Can you work these out from the model? Positions are in its coordinate system, mm. Give positions to 0.01 mm unless a question says otherwise; leave off trailing zeros. Order: outer loops, then holes, each group sorted by start corner. A loop starts at its lowest first (then second) coordinate and runs counter-clockwise, first axis right, second up.
Item 1: If I drill on line 1 along X through (y, z) = (2.25, 101.6); line 2 along X through (y, z) = (4.25, 222); line 3 along X through (y, z) = (2.5, 116.5), over which ranges is the centre line in solid material (lowest first)?
Item 2: I want a section at B-B, the plane y = 2.2. Write out the boundary of the cut face in (x, z), then the cut area to 3 significant figures.
Item 3: I want a section at A-A, the plane z = 101.6. Write out the boundary of the cut face in (x, y), then the cut area to 3 significant figures.
Item 4: I'm going to push flat-ended pins straight in: pin 1 Ø1.4 at (y, z) = (5.5, 125) entering from -X; pin 2 Ø0.6 at (y, z) = (5.5, 123) entering from +X; pin 3 Ø1.4 at (y, z) = (5.5, 124.5) entering from +X; pin 4 Ø9 at (x, z) = (0, 101.6) entering from +Y. Where does each tip first touch, or does it pass through?
Item 5: If we mould it in two halves opening along Z, with no side actions, what happens to faces 1 (the flat face through (1, 0, 175)), 2 (the flat face through (6, 4.724, 121)), 3 (the flat face through (-1, 3, 0))? For each: +Z half, -Z half, draft (parallel to the pull), parting line (faces both ways), or undercut.
Item 6: I want a section at D-D, the plane z = 243. Write out the boundary of the cut face in (x, y).
Item 7: I want a section at C-C, the plane z = 174.5. Write out the boundary of the cut face in (x, y), then the cut area to 3 significant figures.
```python
from build123d import *

# Parameters (mm, degrees)
BOSS_EXTRUDE1_DEPTH = 5.9944
SKETCH2_R           = 5.08
CUT_EXTRUDE1_DEPTH  = 368.170623747
CUT_EXTRUDE2_DEPTH  = 1.27
FILLET1_R           = 6.35


with BuildPart() as part:
    # Sketch1 → Boss-Extrude1 (new body)
    with BuildSketch(Plane(origin=(0, 0, 0), x_dir=(1, 0, 0), z_dir=(0, 1, 0))):
        Polygon((-67.945, 0), (67.945, 0), (91.252255377, -355.6), (-91.252255377, -355.6), align=None)
    extrude(amount=BOSS_EXTRUDE1_DEPTH)

    # Sketch2 → Cut-Extrude1 (cut, through all)
    with BuildSketch(Plane(origin=(0, 5.9944, 0), x_dir=(1, 0, 0), z_dir=(0, 1, 0))):
        with Locations(Location((0, -101.6, 0), (0, 0, 270))):
            Circle(SKETCH2_R)
    extrude(amount=-CUT_EXTRUDE1_DEPTH, mode=Mode.SUBTRACT)

    # Sketch3 → Cut-Extrude2 (cut)
    # profile 1 of 2: a face of its own
    with BuildSketch(Plane(origin=(0, 5.9944, 0), x_dir=(1, 0, 0), z_dir=(0, 1, 0))):
        Polygon((-0.64745098, -123.339411765), (-2.041960784, -123.339411765), (-2.041960784, -125.73), (-2.838823529, -125.73), (-2.838823529, -123.339411765), (-7.420784314, -123.339411765), (-7.420784314, -122.54254902), (-2.676960784, -115.769215686), (-2.041960784, -115.769215686), (-2.041960784, -122.54254902), (-0.64745098, -122.54254902), align=None)
        Polygon((-2.838823529, -122.54254902), (-2.838823529, -117.185514706), (-6.589681373, -122.54254902), align=None, mode=Mode.SUBTRACT)
    # profile 2 of 2: a face of its own
    with BuildSketch(Plane(origin=(0, 5.9944, 0), x_dir=(1, 0, 0), z_dir=(0, 1, 0))):
        with BuildLine():
            add(Edge.make_bspline(
                [(2.583578431, -120.288921569), (2.469757768, -120.233881465), (2.249012298, -120.12713588), (1.956518664, -119.921342429), (1.702152679, -119.699076506), (1.501146738, -119.44377738), (1.338617892, -119.168616459), (1.228149162, -118.865639865), (1.155782886, -118.539856671), (1.148992832, -118.313778727), (1.145490196, -118.197156863)],
                knots=[0, 0, 0, 0, 1.121505956, 2.175065151, 3.167266929, 4.111724904, 5.049364576, 5.994542137, 6.965488487, 8, 8, 8, 8], degree=3))
            add(Edge.make_bspline(
                [(1.145490196, -118.197156863), (1.150650446, -118.072365116), (1.160750204, -117.828119903), (1.228851738, -117.472785505), (1.349283719, -117.141800757), (1.514672213, -116.835914328), (1.722446411, -116.558323216), (1.961706137, -116.307792449), (2.237618257, -116.091502351), (2.542166789, -115.903299875), (2.878819269, -115.755673627), (3.240549794, -115.643784068), (3.628448984, -115.583063263), (3.894888198, -115.574417097), (4.031004902, -115.57)],
                knots=[0, 0, 0, 0, 1.029797524, 2.015542871, 2.97168719, 3.925682005, 4.874436321, 5.825197768, 6.775997772, 7.759919145, 8.771905717, 9.801204739, 10.876694018, 12, 12, 12, 12], degree=3))
            add(Edge.make_bspline(
                [(4.031004902, -115.57), (4.168265453, -115.573915681), (4.437144184, -115.581586081), (4.826482227, -115.649360813), (5.193306386, -115.752803643), (5.528540282, -115.908692567), (5.837903626, -116.092702905), (6.1102298, -116.31471085), (6.35377186, -116.560126292), (6.554706316, -116.839931798), (6.724312123, -117.141452673), (6.837039409, -117.474041466), (6.912766198, -117.827458116), (6.919373101, -118.072230943), (6.922745098, -118.197156863)],
                knots=[0, 0, 0, 0, 1.129990317, 2.213530109, 3.246876235, 4.260696229, 5.250296002, 6.204863837, 7.14791721, 8.090040244, 9.034951547, 9.986644228, 10.972433637, 12, 12, 12, 12], degree=3))
            add(Edge.make_bspline(
                [(6.922745098, -118.197156863), (6.919216595, -118.313762788), (6.912376396, -118.539809833), (6.840365414, -118.865811955), (6.728782095, -119.16750517), (6.571087227, -119.445784939), (6.365570739, -119.697892228), (6.112007529, -119.921560928), (5.819142842, -120.127075675), (5.598450258, -120.233860983), (5.484656863, -120.288921569)],
                knots=[0, 0, 0, 0, 1.034356649, 2.00515765, 2.950193721, 3.883105322, 4.833207204, 5.825260452, 6.878661931, 8, 8, 8, 8], degree=3))
            add(Edge.make_bspline(
                [(5.484656863, -120.288921569), (5.629584904, -120.345274008), (5.909015189, -120.453925018), (6.287487251, -120.674211509), (6.609031926, -120.93355376), (6.873327893, -121.233567804), (7.075041903, -121.576427985), (7.218061472, -121.958672451), (7.307398658, -122.379704945), (7.316483523, -122.673858557), (7.321176471, -122.825808824)],
                knots=[0, 0, 0, 0, 1.104307536, 2.129173671, 3.099289652, 4.029922044, 4.956040619, 5.91100379, 6.920891952, 8, 8, 8, 8], degree=3))
            add(Edge.make_bspline(
                [(7.321176471, -122.825808824), (7.318321613, -122.949426035), (7.312758231, -123.190324178), (7.265802022, -123.539824084), (7.187729342, -123.864910338), (7.08225254, -124.169001718), (6.941227364, -124.448040534), (6.773245337, -124.7078841), (6.567526726, -124.937879056), (6.337999195, -125.1468091), (6.085093931, -125.326864216), (5.825207776, -125.49131202), (5.550637227, -125.624540533), (5.268662499, -125.738439853), (4.972715633, -125.821171296), (4.668146304, -125.883957252), (4.352586022, -125.922213573), (4.139017278, -125.926863823), (4.031004902, -125.929215686)],
                knots=[0, 0, 0, 0, 1.165158113, 2.270593413, 3.316967265, 4.313258111, 5.297614584, 6.258105811, 7.221631145, 8.198179015, 9.17849254, 10.144943439, 11.094310651, 12.051658199, 13.00840578, 13.986862741, 14.981855988, 16, 16, 16, 16], degree=3))
            add(Edge.make_bspline(
                [(4.031004902, -125.929215686), (3.875058258, -125.925696781), (3.571935445, -125.918856875), (3.134122695, -125.846848764), (2.72518677, -125.740751294), (2.34901118, -125.583969435), (2.003278658, -125.380987257), (1.698555205, -125.12058817), (1.419046499, -124.819504607), (1.183989068, -124.46822424), (0.986969857, -124.087207102), (0.851225779, -123.680518964), (0.762222762, -123.259231693), (0.752157029, -122.971528144), (0.747058824, -122.825808824)],
                knots=[0, 0, 0, 0, 1.105131574, 2.1481103, 3.138917951, 4.095657432, 5.029651657, 5.970060793, 6.928497124, 7.934844507, 8.958454957, 9.961540876, 10.967538361, 12, 12, 12, 12], degree=3))
            add(Edge.make_bspline(
                [(0.747058824, -122.825808824), (0.750958552, -122.681150729), (0.75854413, -122.399768191), (0.842695471, -121.995459368), (0.973276047, -121.622346822), (1.158365157, -121.279786493), (1.410049218, -120.969502557), (1.737856358, -120.703220915), (2.131081537, -120.465798713), (2.427881476, -120.34978217), (2.583578431, -120.288921569)],
                knots=[0, 0, 0, 0, 1.026535231, 1.996771007, 2.920245165, 3.827596735, 4.74995178, 5.739273443, 6.81405554, 8, 8, 8, 8], degree=3))
        make_face()
        with BuildLine():
            add(Edge.make_bspline(
                [(6.125882353, -118.228284314), (6.123712551, -118.138717354), (6.119482737, -117.964115492), (6.062504916, -117.712266336), (5.98038969, -117.47610598), (5.859680999, -117.260408538), (5.712107035, -117.063654994), (5.541353334, -116.884667003), (5.342009506, -116.731408764), (5.12047127, -116.600704242), (4.877544231, -116.494065356), (4.612645581, -116.419299497), (4.328142503, -116.37607471), (4.131800472, -116.369987645), (4.031004902, -116.366862745)],
                knots=[0, 0, 0, 0, 1.025357551, 1.998832358, 2.947617169, 3.885211583, 4.820763882, 5.76355694, 6.713535567, 7.695415045, 8.708191046, 9.748023335, 10.843908909, 12, 12, 12, 12], degree=3))
            add(Edge.make_bspline(
                [(4.031004902, -116.366862745), (3.930115428, -116.369479246), (3.734451772, -116.374553651), (3.45109005, -116.424626768), (3.184332955, -116.495249758), (2.942679865, -116.608198219), (2.718840309, -116.735817229), (2.525804645, -116.895504967), (2.351663826, -117.06954252), (2.205860677, -117.266948572), (2.084614049, -117.480848146), (2.006076015, -117.716918532), (1.948805302, -117.966145907), (1.944532402, -118.139739939), (1.942352941, -118.228284314)],
                knots=[0, 0, 0, 0, 1.159100913, 2.247944337, 3.301963364, 4.322203238, 5.306638987, 6.257145066, 7.193841607, 8.131829567, 9.071864958, 10.007877085, 10.983886281, 12, 12, 12, 12], degree=3))
            add(Edge.make_bspline(
                [(1.942352941, -118.228284314), (1.949031284, -118.351609409), (1.962012851, -118.591332492), (2.078543183, -118.932570023), (2.275975601, -119.230977841), (2.538899021, -119.489874585), (2.859494616, -119.695110648), (3.219184028, -119.847237085), (3.614969422, -119.934652524), (3.889465343, -119.946589818), (4.031004902, -119.952745098)],
                knots=[0, 0, 0, 0, 0.976469849, 1.898091887, 2.820632736, 3.792824454, 4.804409425, 5.822739039, 6.877329201, 8, 8, 8, 8], degree=3))
            add(Edge.make_bspline(
                [(4.031004902, -119.952745098), (4.173676734, -119.947027996), (4.449626377, -119.935970226), (4.845443805, -119.843138475), (5.205858473, -119.692440852), (5.5262161, -119.485656096), (5.792340565, -119.229006795), (5.989565911, -118.929321811), (6.105911534, -118.589249373), (6.119116744, -118.350570163), (6.125882353, -118.228284314)],
                knots=[0, 0, 0, 0, 1.129790696, 2.185191953, 3.202539324, 4.213148559, 5.190270146, 6.111921147, 7.032654223, 8, 8, 8, 8], degree=3))
        make_face(mode=Mode.SUBTRACT)
        with BuildLine():
            add(Edge.make_bspline(
                [(6.524313725, -122.891176471), (6.520920106, -122.784069548), (6.514346152, -122.576587224), (6.457940803, -122.276145516), (6.360243009, -122.001268427), (6.229636966, -121.747680515), (6.058383341, -121.524547206), (5.861403172, -121.319861355), (5.625352542, -121.150730147), (5.361894512, -121.006677276), (5.069527463, -120.890509463), (4.748625434, -120.807841497), (4.399931987, -120.756977985), (4.158809369, -120.752120035), (4.034117647, -120.749607843)],
                knots=[0, 0, 0, 0, 1.039609951, 2.013881847, 2.953999013, 3.864434323, 4.771294027, 5.676192345, 6.613334877, 7.578339998, 8.586868343, 9.659784589, 10.789804577, 12, 12, 12, 12], degree=3))
            add(Edge.make_bspline(
                [(4.034117647, -120.749607843), (3.909429768, -120.752131017), (3.668314581, -120.757010204), (3.319569101, -120.807725005), (2.99791307, -120.891154926), (2.704071746, -121.0060513), (2.440098851, -121.149817241), (2.206601469, -121.320933406), (2.00975895, -121.524422815), (1.838623351, -121.747713983), (1.707985337, -122.001259134), (1.610296441, -122.276148125), (1.553888608, -122.576586511), (1.547315006, -122.784069305), (1.543921569, -122.891176471)],
                knots=[0, 0, 0, 0, 1.210068076, 2.339969154, 3.412772499, 4.430563009, 5.395466584, 6.324404951, 7.229208048, 8.135972324, 9.046311831, 9.98633007, 10.960499445, 12, 12, 12, 12], degree=3))
            add(Edge.make_bspline(
                [(1.543921569, -122.891176471), (1.544985709, -122.975375962), (1.547058013, -123.139345961), (1.584332291, -123.377568996), (1.635643144, -123.60328801), (1.710828263, -123.816382724), (1.807662765, -124.01525168), (1.923393036, -124.202835216), (2.065441305, -124.372501414), (2.222512089, -124.532765628), (2.401927227, -124.670707654), (2.59105853, -124.797903891), (2.798953829, -124.900320608), (3.020681135, -124.982957849), (3.253996345, -125.05338774), (3.502487363, -125.098599125), (3.763661295, -125.12731722), (3.942730319, -125.130651369), (4.034117647, -125.132352941)],
                knots=[0, 0, 0, 0, 1.068010984, 2.079843423, 3.054621512, 4.004777055, 4.941776883, 5.859399066, 6.795750163, 7.746088411, 8.702980793, 9.664127459, 10.636408857, 11.637286391, 12.667146169, 13.726670379, 14.839813183, 16, 16, 16, 16], degree=3))
            add(Edge.make_bspline(
                [(4.034117647, -125.132352941), (4.125501134, -125.13064464), (4.304562631, -125.127297307), (4.56680524, -125.098562307), (4.815810816, -125.052774976), (5.050277608, -124.987318412), (5.270990902, -124.903366885), (5.475354786, -124.796869735), (5.667389124, -124.674485413), (5.845554591, -124.535609475), (6.002838181, -124.375684848), (6.144831297, -124.205929646), (6.260573544, -124.018369128), (6.357414326, -123.819495237), (6.432561156, -123.606396774), (6.484253282, -123.379696319), (6.520966694, -123.140347845), (6.523182823, -122.975367067), (6.524313725, -122.891176471)],
                knots=[0, 0, 0, 0, 1.159544989, 2.272071989, 3.343950718, 4.369611888, 5.357637803, 6.335341631, 7.288798869, 8.245161887, 9.194974397, 10.130807493, 11.047922037, 11.984403507, 12.934033413, 13.908272243, 14.932579852, 16, 16, 16, 16], degree=3))
        make_face(mode=Mode.SUBTRACT)
    extrude(amount=-CUT_EXTRUDE2_DEPTH, mode=Mode.SUBTRACT)

    # Fillet1
    fillet1_edges = [part.edges().sort_by_distance(p)[0] for p in [
        (91.252255377, 2.9972, 355.6),
        (-91.252255377, 2.9972, 355.6),
        (-67.945, 2.9972, 0),
        (67.945, 2.9972, 0),
    ]]
    fillet(fillet1_edges, radius=FILLET1_R)


solid = part.part
```
Results list:
1. line 1: x = -74.6 to -5.08, 5.08 to 74.6
1. line 2: x = -82.5 to 82.5
1. line 3: x = -75.58 to 75.58
2. outline: (-90.81, 348.83) - (-68.33, 5.93) arc R6.35 ccw to (-62, 0) - (62, 0) arc R6.35 ccw to (68.33, 5.93) - (90.81, 348.83) arc R6.35 ccw to (84.47, 355.6) - (-84.47, 355.6) arc R6.35 ccw to start; hole circle Ø10.16 at (0, 101.6)
2. area: 56,500 mm2
3. outline: (-74.6, 0) - (-5.08, 0) - (-5.08, 5.99) - (-74.6, 5.99) - close; (5.08, 0) - (74.6, 0) - (74.6, 5.99) - (5.08, 5.99) - close
3. area: 834 mm2
4. pin 1: stops at x = -76.18
4. pin 2: stops at x = 76.03
4. pin 3: stops at x = 76.15
4. pin 4: passes through
5. face 1: draft
5. face 2: undercut
5. face 3: -Z half
6. outline: (-83.87, 0) - (83.87, 0) - (83.87, 5.99) - (-83.87, 5.99) - close
7. outline: (-79.38, 0) - (79.38, 0) - (79.38, 5.99) - (-79.38, 5.99) - close
7. area: 952 mm2
